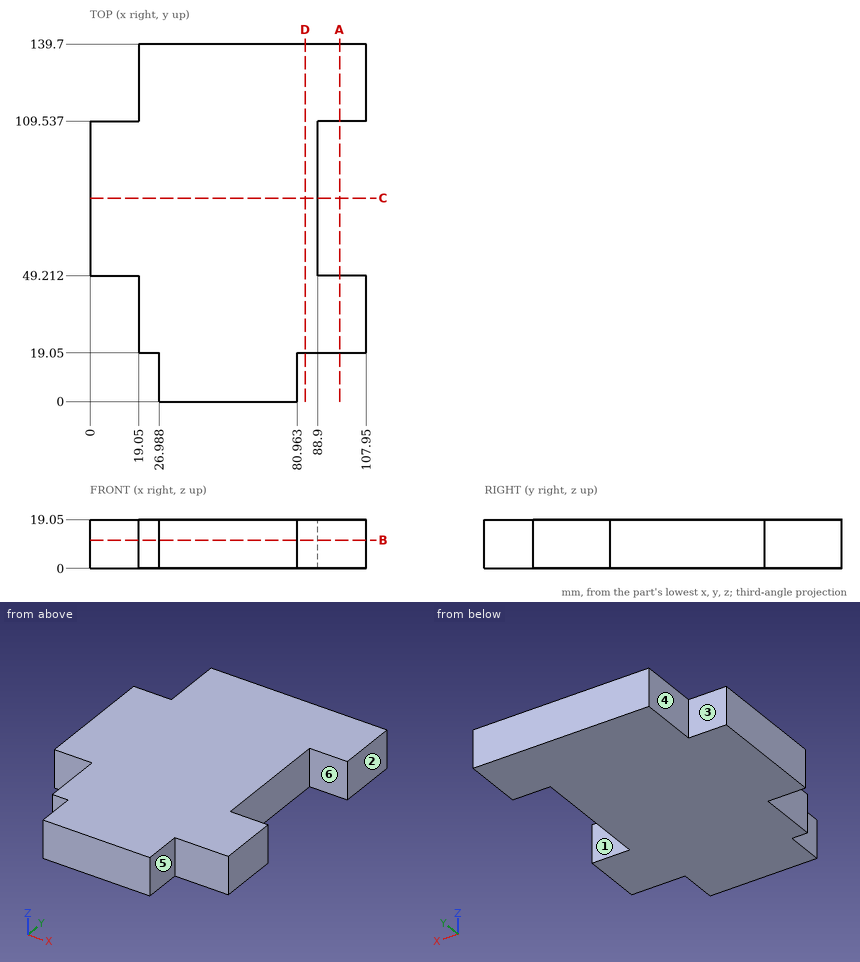
Drawing for the job (mm, zero at the part's lowest x, y, z). A direction names the side the tool comes from. Round coordinates to 2 decimals unless told otherwise and drop trailing zeros. Write each loop counter-clockwise with the first axis right and the second up, starting at its lowest first coordinate (ties: lowest second). Pieces come first, ordered by that corner, then holes.
Item 1: Mould opens along Y. For the marked faces 1, 2 and 3 say: released by +Y, released by -Y, zero draft, split by the parting line, or undercut.
Filled in:
face 1: undercut
face 2: zero draft
face 3: released by +Y
Item 2: Band-saw the part on D-D on x = 84. Write the cut outline in (y, z).
Filled in:
outline: (19.05, 0) - (139.7, 0) - (139.7, 19.05) - (19.05, 19.05) - close
Item 3: Band-saw the part on A-A on x = 97.5. Write the cut outline in (y, z), then the cut area to 3 significant figures.
Filled in:
outline: (19.05, 0) - (49.21, 0) - (49.21, 19.05) - (19.05, 19.05) - close; (109.54, 0) - (139.7, 0) - (139.7, 19.05) - (109.54, 19.05) - close
area: 1,150 mm2
Item 4: Tool access for the marked faces 4, 5 and 6: list every direction of +Z, -Z, +X, -X, +Y, -Y with a clear straight run to the whole face (end or side of a thin tool).
Filled in:
face 4: +Z, -Z, -X, +Y
face 5: +Z, -Z, +X, -Y
face 6: +Z, -Z, +X
Item 5: Drill centre lines: L1, parallel to Y at x = 97.5, z = 15; L2, parallel to X at y = 45.5, z = 5; L3, parallel to X at y = 103, z = 14. Where is each one in solid material? Low to high.
Filled in:
L1: y = 19.05 to 49.21, 109.54 to 139.7
L2: x = 19.05 to 107.95
L3: x = 0 to 88.9
Item 6: Band-saw the part on C-C on y = 79.5. Write the cut outline in (x, z), then the cut area to 3 significant figures.
Filled in:
outline: (0, 0) - (88.9, 0) - (88.9, 19.05) - (0, 19.05) - close
area: 1,690 mm2
Item 7: Band-saw the part on B-B on z = 11. Write the cut outline in (x, y).
Filled in:
outline: (0, 49.21) - (19.05, 49.21) - (19.05, 19.05) - (26.99, 19.05) - (26.99, 0) - (80.96, 0) - (80.96, 19.05) - (107.95, 19.05) - (107.95, 49.21) - (88.9, 49.21) - (88.9, 109.54) - (107.95, 109.54) - (107.95, 139.7) - (19.05, 139.7) - (19.05, 109.54) - (0, 109.54) - close
Item 8: Drop flat-ended pins along their axis: pin 1 Ø5 at (y, z) = (15, 16.5) entering from -X; pin 2 Ø5.5 at (x, z) = (103, 9.5) entering from -Y; pin 3 Ø9.5 at (y, z) = (37, 6.5) entering from -X. Give the stop position or say it passes through.
Filled in:
pin 1: stops at x = 26.99
pin 2: stops at y = 19.05
pin 3: stops at x = 19.05
